Autodesk Inventor part; units mm, degrees
ref_plane "Work Plane1" through (8.75, -15.1554, 14.75) normal (0.866, 0.5, 0) x (0, 0, -1)
ref_plane "YZ Plane" through (0, 0, 0) normal (1, 0, 0) x (0, 1, 0)
ref_plane "XZ Plane" through (0, 0, 0) normal (0, 1, 0) x (-1, 0, 0)
sketch "Sketch1" plane through (0, 0, 0) normal (0, 0, 1) x (1, 0, 0)
  circle A0 centre (0, 0) radius 35
  circle A1 centre (0, 0) radius 4.5
  dimension "d0" = 70
  dimension "d1" = 9
extrude "Extrusion1" add sketch "Sketch1" along normal blind 14.75
sketch "Sketch2" plane through (0, 0, 14.75) normal (0, 0, 1) x (1, 0, 0)
  circle A0 centre (0, 0) radius 13.5
  dimension "d4" = 27
extrude "Extrusion2" cut sketch "Sketch2" against normal blind 8
sketch "Sketch3" plane through (0, 0, 6.75) normal (0, 0, 1) x (1, 0, 0)
  circle A0 centre (0, 0) radius 7.5
  dimension "d7" = 15
extrude "Extrusion3" cut sketch "Sketch3" against normal blind 5
sketch "Sketch4" plane through (0, 0, 6.75) normal (0, 0, 1) x (1, 0, 0)
  circle A0 centre (9.525, 0) radius 1.5
  circle A1 centre (4.7625, 8.2489) radius 1.5
  circle A2 centre (-4.7625, 8.2489) radius 1.5
  circle A3 centre (-9.525, 0) radius 1.5
  circle A4 centre (-4.7625, -8.2489) radius 1.5
  circle A5 centre (4.7625, -8.2489) radius 1.5
  point P0 (0, 0)
  dimension "d10" = 3
  dimension "d11" = 9.525
  dimension "d14" = 360
extrude "Extrusion4" cut sketch "Sketch4" against normal through all
sketch "Sketch5" plane through (0, 0, 14.75) normal (0, 0, 1) x (1, 0, 0)
  circle A0 centre (23, 0) radius 2.5
  circle A1 centre (11.5, 19.9186) radius 2.5
  circle A2 centre (-11.5, 19.9186) radius 2.5
  circle A3 centre (-23, 0) radius 2.5
  circle A4 centre (-11.5, -19.9186) radius 2.5
  circle A5 centre (11.5, -19.9186) radius 2.5
  point P0 (0, 0)
  dimension "d18" = 5
  dimension "d19" = 23
  dimension "d22" = 360
extrude "Extrusion5" cut sketch "Sketch5" against normal through all contours A2 | A3 | A4 | A5
sketch "Sketch7" plane through (0, 0, 14.75) normal (0, 0, 1) x (1, 0, 0)
  line L0 (17.5, 30.3109) -> (22.6962, 33.3109)
  line L1 (22.6962, 33.3109) -> (40.1962, 3)
  line L2 (40.1962, 3) -> (35, 0)
  line L3 (35, 0) -> (17.5, 30.3109)
  circle A0 centre (0, 0) radius 35 construction
  line L4 (0, 0) -> (26.25, 15.1554)
  line L5 (0, 0) -> (26.25, 0)
  dimension "d33" = 6
  dimension "d34" = 35
  dimension "d43" = 30
extrude "Extrusion7" add sketch "Sketch7" against normal blind 14.75
sketch "Sketch8" plane through (40.1962, 3, 14.75) normal (0.866, 0.5, 0) x (0, 0, -1)
  circle A0 centre (7.375, 30) radius 2.5
  circle A1 centre (7.375, 5) radius 2.5
  line L0 (7.375, 30) -> (7.375, 5) construction
  line L1 (14.75, 35) -> (14.75, 0)
  line L2 (0, 35) -> (14.75, 35)
  point P0 (14.75, 17.5)
  point P1 (14.75, 17.5)
  point P2 (7.375, 17.5)
  point P3 (7.375, 35)
  dimension "d37" = 5
  dimension "d38" = 5
  dimension "d39" = 25
extrude "Extrusion8" cut sketch "Sketch8" against normal blind 25
sketch "Sketch9" plane through (40.1962, 3, 14.75) normal (0.866, 0.5, 0) x (0, 0, -1)
  circle A0 centre (7.375, 17.5) radius 3
  line L0 (14.75, 35) -> (14.75, 0)
  circle A1 centre (7.375, 30) radius 2.5 construction
  point P0 (14.75, 17.5)
  point P1 (14.75, 17.5)
  dimension "d42" = 6
extrude "Extrusion9" cut sketch "Sketch9" against normal through all
ref_plane "Work Plane1" through (8.75, -15.1554, 14.75) normal (0.866, 0.5, 0) x (0, 0, -1)
sketch "Sketch11" plane through (8.75, -15.1554, 14.75) normal (0.866, 0.5, 0) x (0, 0, -1)
  line L0 (13, 22) -> (13, 13)
  line L1 (13, 10) -> (13, 25)
  line L2 (0, 35) -> (0, 0)
  line L3 (0, 35) -> (0, 0)
  line L4 (0, 4) -> (0, 31)
  line L5 (13, 10) -> (13, 25)
  line L6 (13, 20.5) -> (3, 20.5)
  line L7 (3, 20.5) -> (3, 14.5)
  line L8 (3, 14.5) -> (13, 14.5)
  line L9 (13, 14.5) -> (13, 20.5)
  point P0 (14.75, 17.5)
  point P1 (0, -0.5)
  point P2 (0, 12.5)
  point P3 (0, 34)
  point P4 (0, 47)
  point P5 (0, -0.5)
  point P6 (0, 12.5)
  point P7 (0, 22.5)
  point P8 (0, 35.5)
  point P9 (0, 22.5)
  point P10 (0, 35.5)
  point P11 (0, -12)
  point P12 (0, 1)
  point P13 (8, 20.4342)
  point P14 (8, 14.5658)
  dimension "d47" = 3
extrude "Extrusion10" cut sketch "Sketch11" against normal through all
sketch "Sketch12" plane through (0, 0, 14.75) normal (0, 0, 1) x (1, 0, 0)
  arc A0 (17.5, 30.3109) -> (35, 0) centre (0, 0) ccw
  circle A1 centre (0, 0) radius 35
  circle A2 centre (0, 0) radius 31
  dimension "d50" = 4
extrude "Extrusion11" cut sketch "Sketch12" against normal blind 5 contours A2
sketch "Sketch13" plane through (0, 0, 9.75) normal (0, 0, 1) x (1, 0, 0)
  line L0 (7.3577, 23.8779) -> (11.8577, 16.0836)
  line L1 (11.8577, 16.0836) -> (16.1878, 18.5836)
  line L2 (16.1878, 18.5836) -> (11.6878, 26.3779)
  line L3 (11.6878, 26.3779) -> (7.3577, 23.8779)
  line L4 (3.1552, 17.1568) -> (3.9358, 15.8047)
  line L5 (17.6181, 25.5069) -> (3.1552, 17.1568)
  line L6 (3.5455, 16.4808) -> (9.6077, 19.9808)
  circle A0 centre (0, 0) radius 4.5
  line L7 (0, 0) -> (38.9378, 22.4808)
  line L8 (0, 0) -> (44.9615, 0) construction
  line L9 (24.3577, -5.567) -> (19.8577, 2.2272)
  line L10 (19.8577, 2.2272) -> (24.1878, 4.7272)
  line L11 (24.1878, 4.7272) -> (28.6878, -3.067)
  line L12 (28.6878, -3.067) -> (24.3577, -5.567)
  line L13 (16.4358, -5.8459) -> (15.6552, -4.4938)
  line L14 (30.8987, 2.5042) -> (16.4358, -5.8459)
  line L15 (16.0455, -5.1699) -> (22.1077, -1.6699)
  point P0 (30.8987, 2.5042)
  point P1 (22.1077, -1.6699)
  dimension "d54" = 5
  dimension "d56" = 9
  dimension "d59" = 7
  dimension "d60" = 30
extrude "Extrusion12" cut sketch "Sketch13" against normal blind 7.45 contours L0 L5 L2 L1 | L0 L3 L2 L5 | L9 L10 L11 L14 | L14 L11 L12 L9
properties part number "AA046" material "ABS Plastic"
Part model, mm, in its own coordinate system. A direction names the side the tool comes from. Give positions to 0.01 mm unless a question says otherwise; leave off trailing zeros. Loops run counter-clockwise (first coordinate to the right, second up) from the corner with the lowest first, then second, coordinate; pieces in that order, holes last.
(1) Band-saw the part on B-B (z = 13.5). Write the cut outline in (x, y), and give its area (3 significant figures).
Return value:
outline: (17.5, 30.31) arc R35 ccw (long way) to (35, 0) - (40.2, 3) - (22.7, 33.31) - close; hole circle Ø62 at (0, 0)
area: 928 mm2
(2) Band-saw the part on A-A (x = 0). Write the cut outline in (y, z).
Return value:
outline: (-35, 0) - (-4.5, 0) - (-4.5, 1.75) - (-7.5, 1.75) - (-7.5, 6.75) - (-13.5, 6.75) - (-13.5, 9.75) - (-31, 9.75) - (-31, 14.75) - (-35, 14.75) - close; (4.5, 0) - (35, 0) - (35, 14.75) - (31, 14.75) - (31, 9.75) - (13.5, 9.75) - (13.5, 6.75) - (7.5, 6.75) - (7.5, 1.75) - (4.5, 1.75) - close
(3) Drill centre lines: line 1 along Y through (x, z) = (0, 9.5); line 2 along Y through (x, z) = (3.5, 6); line 3 along X through (y, z) = (10, 8). Where is each one in solid material? Low to high.
Return value:
line 1: y = -35 to -13.5, 13.5 to 35
line 2: y = -34.82 to -9.06, -7.44 to -6.63, 6.63 to 7.44, 9.06 to 16.56, 18.87 to 34.82
line 3: x = -33.54 to -9.07, 9.07 to 11.45, 23.19 to 36.15
(4) Pin check, flat tips, straight feed: pin 1 (5 mm diameter, centred on x = -16.5, y = -22, fed in from +Z); pin 2 (5 mm diameter, centred on x = 4.76, y = 8.25, fed in from +Z); pin 3 (1 mm diameter, centred on y = 12, z = 4, fed in from -X); pin 4 (2.5 mm diameter, centred on x = 9.525, y = 0, fed in from -Z). Stop position of each tip, or through.
Return value:
pin 1: stops at z = 9.75
pin 2: stops at z = 6.75
pin 3: stops at x = -33.06
pin 4: passes through
(5) 3-axis set-ups, long thin cutter, end or side, ignore diameter. For faces 5 (the cylindrical face through (-8.139, -0.575, 3.422)), 6 (the flat face through (13.992, 17.316, 6.077)), 7 (the flat face through (16.026, -5.141, 7.347)): which of +Z, -Z, +X, -X, +Y, -Y reach the whole face in a straight line?
Return value:
face 5: +Z, -Z
face 6: +Z
face 7: none
(6) Pull direction Y, two halves, no side cores. Call faces 1 (the flat face through (-9, 14, 9.75)), 2 (the cylindrical face through (6.634, 3.499, 3.729)), 3 (the cylindrical face through (-29.65, -18.6, 12.19)), 4 (the flat face through (20.06, 31.79, 7.48)): pulls with the +Y half, pulls with the -Y half, needs draft (parallel to the pull), parting line crosses it, or undercut.
Return value:
face 1: undercut
face 2: undercut
face 3: parting line crosses it
face 4: pulls with the +Y half
